```python
from build123d import *

# Parameters (mm, degrees)
BOSS_EXTRUDE1_DEPTH      = 1.5
BOSS_EXTRUDE1_DEPTH_BACK = 1.5
BOSS_EXTRUDE2_DEPTH      = 1.5
BOSS_EXTRUDE2_DEPTH_BACK = 1.5
SKETCH6_W                = 9.75
SKETCH6_H                = 3
SKETCH6_W_2              = 0.965
SKETCH6_H_2              = 1.5
BOSS_EXTRUDE4_DEPTH      = 2.5
CUT_EXTRUDE1_DEPTH       = 1.5
SKETCH11_R               = 1.4
CUT_EXTRUDE2_DEPTH       = 60.213596412
SKETCH13_R               = 10.5
BOSS_EXTRUDE5_DEPTH      = 2
BOSS_EXTRUDE5_DEPTH_BACK = 5
CUT_EXTRUDE3_DEPTH       = 10
CUT_EXTRUDE3_DEPTH_BACK  = 10
SKETCH15_R               = 9
CUT_EXTRUDE4_DEPTH       = 10
CUT_EXTRUDE5_DEPTH       = 4.1
SKETCH19_R               = 8.75
CUT_EXTRUDE6_DEPTH       = 2.5
SKETCH23_R               = 1.75
CUT_EXTRUDE9_DEPTH       = 10


with BuildPart() as part:
    # Sketch1 → Revolve1 (revolve)
    with BuildSketch(Plane.XY, mode=Mode.PRIVATE) as revolve1_sk:
        with BuildLine():
            Line((-20.885, 0), (-20.885, 11.793939121))
            ThreePointArc((-20.885, 11.793939121), (-12.091372858, 20.714220415), (0, 23.985))
            Line((0, 23.985), (0, 25.485))
            ThreePointArc((0, 25.485), (-18.020616319, 18.020616319), (-25.485, 0))
            Line((-25.485, 0), (-24.285, 0))
            Line((-24.285, 0), (-24.285, 0.5))
            Line((-24.285, 0.5), (-22.085, 0.5))
            Line((-22.085, 0.5), (-22.085, 0))
            Line((-22.085, 0), (-20.885, 0))
        make_face()
    revolve(revolve1_sk.sketch.rotate(Axis((0, 0, 0), (0, 1, 0)), 270), axis=Axis((0, 0, 0), (0, 1, 0)))



with BuildPart() as body_2:
    # Sketch2 → Boss-Extrude1 (new, two sides)
    with BuildSketch(Plane.XY) as boss_extrude1_sk:
        with BuildLine():
            Line((-24.9, 0), (-35, 0))
            ThreePointArc((-35, 0), (0, 35), (35, 0))
            Line((35, 0), (24.9, 0))
            ThreePointArc((24.9, 0), (0, 24.9), (-24.9, 0))
        make_face()
    extrude(amount=BOSS_EXTRUDE1_DEPTH)
    extrude(boss_extrude1_sk.sketch, amount=-BOSS_EXTRUDE1_DEPTH_BACK)

    # Sketch3 → Boss-Extrude2 (add, two sides)
    with BuildSketch(Plane(origin=(0, 0, 0), x_dir=(0, 0, -1), z_dir=(1, 0, 0))) as boss_extrude2_sk:
        with BuildLine():
            Line((35, 0), (24.9, 0))
            ThreePointArc((24.9, 0), (0, 24.9), (-24.9, 0))
            Line((-24.9, 0), (-35, 0))
            ThreePointArc((-35, 0), (0, 35), (35, 0))
        make_face()
    extrude(amount=BOSS_EXTRUDE2_DEPTH)
    extrude(boss_extrude2_sk.sketch, amount=-BOSS_EXTRUDE2_DEPTH_BACK)


with BuildPart() as part_1:
    add(part.part)

    add(body_2.part)  # Revolve3 merges body 2
    # Sketch6 → Revolve3 (revolve)
    with BuildSketch(Plane(origin=(0, 0, 0), x_dir=(0, 0, -1), z_dir=(1, 0, 0)), mode=Mode.PRIVATE) as revolve3_sk:
        with Locations((30.125, 0)):
            Rectangle(SKETCH6_W, SKETCH6_H)
        with Locations((24.7675, 0.75)):
            Rectangle(SKETCH6_W_2, SKETCH6_H_2)
    revolve(revolve3_sk.sketch.rotate(Axis((0, 0, 0), (0, -1, 0)), 180), axis=Axis((0, 0, 0), (0, -1, 0)))

    # Sketch9 → Cut-Revolve1 (revolve, cut)
    with BuildSketch(Plane.XY, mode=Mode.PRIVATE) as cut_revolve1_sk:
        with BuildLine():
            Line((34.507469645, 5.851028856), (35.470882951, 5.851028856))
            Line((35.470882951, 5.851028856), (35.470882951, 1.5))
            Line((35.470882951, 1.5), (34.96784237, 1.5))
            ThreePointArc((34.96784237, 1.5), (34.805712289, 3.682715312), (34.507469645, 5.851028856))
        make_face()
    revolve(cut_revolve1_sk.sketch.rotate(Axis((0, 0, 0), (0, 1, 0)), 180), axis=Axis((0, 0, 0), (0, 1, 0)), mode=Mode.SUBTRACT)

    # Sketch7 → Boss-Extrude4 (add)
    with BuildSketch(Plane(origin=(0, 1.5, 0), x_dir=(1, 0, 0), z_dir=(0, 1, 0))):
        with BuildLine():
            Line((23.044996888, 10.777909974), (22.609782845, 10.667601403))
            ThreePointArc((22.609782845, 10.667601403), (24.220082694, 6.195772291), (24.954959427, 1.5))
            Line((24.954959427, 1.5), (25.396559314, 1.5))
            Line((25.396559314, 1.5), (34.96784237, 1.5))
            ThreePointArc((34.96784237, 1.5), (31.274568745, 9.053705347), (23.044996888, 10.777909974))
        make_face()
        with BuildLine():
            ThreePointArc((10.667601403, -22.609782845), (6.195772291, -24.220082694), (1.5, -24.954959427))
            Line((1.5, -24.954959427), (1.5, -25.396559314))
            Line((1.5, -25.396559314), (1.5, -34.96784237))
            ThreePointArc((1.5, -34.96784237), (9.053705347, -31.274568745), (10.777909974, -23.044996888))
            Line((10.777909974, -23.044996888), (10.667601403, -22.609782845))
        make_face()
        with BuildLine():
            Line((-25.396559314, -1.5), (-34.96784237, -1.5))
            ThreePointArc((-34.96784237, -1.5), (-31.274568745, -9.053705347), (-23.044996888, -10.777909974))
            Line((-23.044996888, -10.777909974), (-22.609782845, -10.667601403))
            ThreePointArc((-22.609782845, -10.667601403), (-24.220082694, -6.195772291), (-24.954959427, -1.5))
            Line((-24.954959427, -1.5), (-25.396559314, -1.5))
        make_face()
        with BuildLine():
            ThreePointArc((-2.626689255, 34.901296588), (-9.387133949, 30.818973666), (-10.777909974, 23.044996888))
            ThreePointArc((-10.777909974, 23.044996888), (-6.25053836, 24.661021779), (-1.5, 25.396559314))
            Line((-1.5, 25.396559314), (-1.5, 34.96784237))
            ThreePointArc((-1.5, 34.96784237), (-2.063612885, 34.939111349), (-2.626689255, 34.901296588))
        make_face()
        with BuildLine():
            Line((-10.777909974, 23.044996888), (-10.667601403, 22.609782845))
            ThreePointArc((-10.667601403, 22.609782845), (-6.195772291, 24.220082694), (-1.5, 24.954959427))
            Line((-1.5, 24.954959427), (-1.5, 25.396559314))
            ThreePointArc((-1.5, 25.396559314), (-6.25053836, 24.661021779), (-10.777909974, 23.044996888))
        make_face()
    extrude(amount=BOSS_EXTRUDE4_DEPTH)

    # Sketch10 → Cut-Extrude1 (cut)
    with BuildSketch(Plane(origin=(0, 4, 0), x_dir=(1, 0, 0), z_dir=(0, 1, 0))):
        Polygon((4.2, -31.327119097), (6.9, -29.76827337), (6.9, -26.650581916), (4.2, -25.091736189), (1.5, -26.650581916), (1.5, -29.76827337), align=None)
        Polygon((-25.091736189, -4.2), (-26.650581916, -1.5), (-29.76827337, -1.5), (-31.327119097, -4.2), (-29.76827337, -6.9), (-26.650581916, -6.9), align=None)
        Polygon((-4.2, 31.327119097), (-6.9, 29.76827337), (-6.9, 26.650581916), (-4.2, 25.091736189), (-1.5, 26.650581916), (-1.5, 29.76827337), align=None)
        Polygon((31.327119097, 4.2), (29.76827337, 6.9), (26.650581916, 6.9), (25.091736189, 4.2), (26.650581916, 1.5), (29.76827337, 1.5), align=None)
    extrude(amount=-CUT_EXTRUDE1_DEPTH, mode=Mode.SUBTRACT)

    # Sketch11 → Cut-Extrude2 (cut, through all)
    with BuildSketch(Plane(origin=(0, 2.5, 0), x_dir=(1, 0, 0), z_dir=(0, 1, 0))):
        with Locations(Location((28.209427643, 4.2, 0), (0, 0, 270))):
            Circle(SKETCH11_R)
        with Locations(Location((4.2, -28.209427643, 0), (0, 0, 270))):
            Circle(SKETCH11_R)
        with Locations(Location((-28.209427643, -4.2, 0), (0, 0, 270))):
            Circle(SKETCH11_R)
        with Locations(Location((-4.2, 28.209427643, 0), (0, 0, 270))):
            Circle(SKETCH11_R)
    extrude(amount=-CUT_EXTRUDE2_DEPTH, mode=Mode.SUBTRACT)

    # Sketch13 → Boss-Extrude5 (add, two sides)
    with BuildSketch(Plane(origin=(-12.655947457, 12.655947457, 12.655947457), x_dir=(-0.8164965809277261, -0.408248290463863, -0.408248290463863), z_dir=(0.5773502691896257, -0.5773502691896258, -0.5773502691896258))) as boss_extrude5_sk:
        with Locations(Location((0, 0, 0), (0, 0, 270))):
            Circle(SKETCH13_R)
    extrude(amount=BOSS_EXTRUDE5_DEPTH)
    extrude(boss_extrude5_sk.sketch, amount=-BOSS_EXTRUDE5_DEPTH_BACK)

    # Sketch12 → Cut-Extrude3 (cut, two sides)
    with BuildSketch(Plane(origin=(-12.655947457, 12.655947457, 12.655947457), x_dir=(-0.8164965809277261, -0.408248290463863, -0.408248290463863), z_dir=(0.5773502691896257, -0.5773502691896258, -0.5773502691896258))) as cut_extrude3_sk:
        with BuildLine():
            Line((0.352106197, -6.089829327), (5.097893803, -3.349847575))
            ThreePointArc((5.097893803, -3.349847575), (5.282754963, 3.05), (-0.352106197, 6.089829327))
            Line((-0.352106197, 6.089829327), (-5.097893803, 3.349847575))
            ThreePointArc((-5.097893803, 3.349847575), (-5.282754963, -3.05), (0.352106197, -6.089829327))
        make_face()
    extrude(amount=CUT_EXTRUDE3_DEPTH, mode=Mode.SUBTRACT)
    extrude(cut_extrude3_sk.sketch, amount=-CUT_EXTRUDE3_DEPTH_BACK, mode=Mode.SUBTRACT)

    # Sketch15 → Cut-Extrude4 (cut)
    with BuildSketch(Plane(origin=(-11.501246918, 11.501246918, 11.501246918), x_dir=(-0.40824829046386274, 0.40824829046386296, -0.8164965809277264), z_dir=(0.5773502691896258, -0.5773502691896262, -0.5773502691896255))):
        Circle(SKETCH15_R)
    extrude(amount=CUT_EXTRUDE4_DEPTH, mode=Mode.SUBTRACT)

    # Sketch18 → Cut-Extrude5 (cut)
    with BuildSketch(Plane(origin=(-15.542698803, 15.542698803, 15.542698803), x_dir=(0.40824829046386274, -0.40824829046386296, 0.8164965809277264), z_dir=(-0.5773502691896258, 0.5773502691896262, 0.5773502691896255))):
        with BuildLine():
            Line((0.654858953, -7.06973548), (5.795141047, -4.101992229))
            ThreePointArc((5.795141047, -4.101992229), (6.148780367, 3.55), (-0.654858953, 7.06973548))
            ThreePointArc((-0.654858953, 7.06973548), (-3.55, 6.148780367), (-5.795141047, 4.101992229))
            ThreePointArc((-5.795141047, 4.101992229), (-6.148780367, -3.55), (0.654858953, -7.06973548))
        make_face()
    extrude(amount=-CUT_EXTRUDE5_DEPTH, mode=Mode.SUBTRACT)

    # Sketch19 → Cut-Extrude6 (cut)
    with BuildSketch(Plane(origin=(-15.542698803, 15.542698803, 15.542698803), x_dir=(0.40824829046386274, -0.40824829046386296, 0.8164965809277264), z_dir=(-0.5773502691896258, 0.5773502691896262, 0.5773502691896255))):
        with Locations(Location((0, 0, 0), (0, 0, 270))):
            Circle(SKETCH19_R)
    extrude(amount=-CUT_EXTRUDE6_DEPTH, mode=Mode.SUBTRACT)

    # Sketch23 → Cut-Extrude9 (cut)
    with BuildSketch(Plane(origin=(0, 1.5, 0), x_dir=(1, 0, 0), z_dir=(0, 1, 0))):
        with Locations(Location((21.213203436, -21.213203436, 0), (0, 0, 270))):
            Circle(SKETCH23_R)
        with Locations(Location((-21.213203436, 21.213203436, 0), (0, 0, 270))):
            Circle(SKETCH23_R)
    extrude(amount=-CUT_EXTRUDE9_DEPTH, mode=Mode.SUBTRACT)

    # SurfaceCut1
    split(bisect_by=Plane(origin=(0, 0, 0), x_dir=(0, 0, -1), z_dir=(1, 0, 0)), keep=Keep.TOP)


solid = part_1.part
```
Input: part model. Units: mm. Frame: model coordinates. A direction names the side the tool comes from. Round coordinates to 2 decimals unless told otherwise and drop trailing zeros. Order: outer loops, then holes, each group sorted by start corner. A loop starts at its lowest first (then second) coordinate and runs counter-clockwise, first axis right, second up. Notation, with made-up numbers: (-31.75, 38.25) - (21.25, 38.25) arc R32 ccw to (21.25, 75.25) - close; hole circle Ø9 at (-2.5, 42). An arc over 180 degrees is marked (long way). Answer in a Markdown table with one row per item.
Item 1: Reachability of faces 4 (the cylindrical face through (4.26, 0.53, 26.81)), 5 (the flat face through (25, 0, 0)), 6 (the flat face through (18.5, 18.5, 1.5)), 7 (the flat face through (4, 2.5, 30)) from +Z, -Z, +X, -X, +Y, -Y: full face, straight path, thin tool, end or side. Return the list, or none.
Model answer:
| item | result |
|---|---|
| face 4 | +Y, -Y |
| face 5 | -X, -Y |
| face 6 | +Z, +X, +Y |
| face 7 | +Y |
Item 2: Line query: line 1 (X direction, y = 13.5, z = -26.5); line 2 (Z direction, x = 11, y = 30); line 3 (Z direction, x = 16.5, y = 4). Output: solid intervals per line, ascending.
Model answer:
| item | result |
|---|---|
| line 1 | x = 0 to 1.5 |
| line 2 | z = -1.5 to 1.5 |
| line 3 | z = -19.01 to -12.8, 12.8 to 19.01 |
Item 3: Section query B-B (z = -18). Return the cut outline in (x, y), then the cut area to 3 significant figures.
Model answer:
| item | result |
|---|---|
| outline | (0, 15.85) arc R15.85 cw to (10.59, 11.79) - (10.59, 0) - (12.8, 0) - (12.8, 0.5) - (16.3, 0.5) - (16.3, 0) - (17.71, 0) - (17.71, -1.5) - (30.02, -1.5) - (30.02, 1.5) - (17.98, 1.5) arc R18.04 ccw to (1.5, 17.98) - (1.5, 30.02) - (0, 30.02) - close |
| area | 154 mm² |
Item 4: Section query A-A (y = 17). Return the cut outline in (x, z), then the cut area to 3 significant figures.
Model answer:
| item | result |
|---|---|
| outline | (0, -30.59) - (1.5, -30.59) - (1.5, -18.93) arc R18.99 ccw to (18.93, -1.5) - (30.59, -1.5) - (30.59, 1.5) - (18.93, 1.5) arc R18.99 ccw to (1.5, 18.93) - (1.5, 30.59) - (0, 30.59) - (0, 16.92) arc R16.92 cw to (0, -16.92) - close |
| area | 186 mm² |
Item 5: Section query C-C (y = 23). Return the cut outline in (x, z), then the cut area to 3 significant figures.
Model answer:
| item | result |
|---|---|
| outline | (0, -26.38) - (1.5, -26.38) - (1.5, -10.87) arc R10.98 ccw to (10.87, -1.5) - (26.38, -1.5) - (26.38, 1.5) - (10.87, 1.5) arc R10.98 ccw to (1.5, 10.87) - (1.5, 26.38) - (0, 26.38) - (0, 6.8) arc R6.8 cw to (0, -6.8) - close |
| area | 209 mm² |
Item 6: Pin query (flat end, axial travel): pin 1 (11 mm diameter, centred on x = 14.5, z = -5, fed in from -Y); pin 2 (1.5 mm diameter, centred on x = 21, z = -10, fed in from -Y); pin 3 (12 mm diameter, centred on x = 12.5, z = 16.5, fed in from +Y). Return the tip coordinate at first contact, or that it passes through.
Model answer:
| item | result |
|---|---|
| pin 1 | stops at y = 11.88 |
| pin 2 | stops at y = 0.5 |
| pin 3 | stops at y = 20.82 |
Item 7: Section query D-D (z = -30). Return the cut outline in (x, y), then the cut area to 3 significant figures.
Model answer:
| item | result |
|---|---|
| outline | (0, -1.5) - (18.03, -1.5) - (18.03, 1.5) - (1.5, 1.5) - (1.5, 18.03) - (0, 18.03) - close |
| area | 78.9 mm² |
Item 8: Mould query, pull axis X, two halves, no side actions, for faces 1 (the cylindrical face through (0.76, 26.03, 23.4)), 2 (the cylindrical face through (8.98, 2.73, 31.37)), 3 (the cylindrical face through (27.358, 0.528, -5.311)). Classes: released by +X, released by -X, zero draft, split by the parting line, or undercut.
Model answer:
| item | result |
|---|---|
| face 1 | zero draft |
| face 2 | released by +X |
| face 3 | undercut |
